Answer from the drawing. Dimensions are ordinates in mm from the lowest x, y and z of the part. Coordinates: 2 decimals unless noted, no trailing zeros. Write each loop counter-clockwise with the first axis right and the second up, starting at its lowest first coordinate (ties: lowest second). Pieces come first, ordered by that corner, then holes. Notation, with made-up numbers: (-37, 5.25) -> (-17, 5.25) arc R12 ccw to (-17, 9.25) -> close; hole circle Ø9 at (52, -19). An arc over 180 degrees is marked (long way). One line per item, written item: value. Start each with the question number.
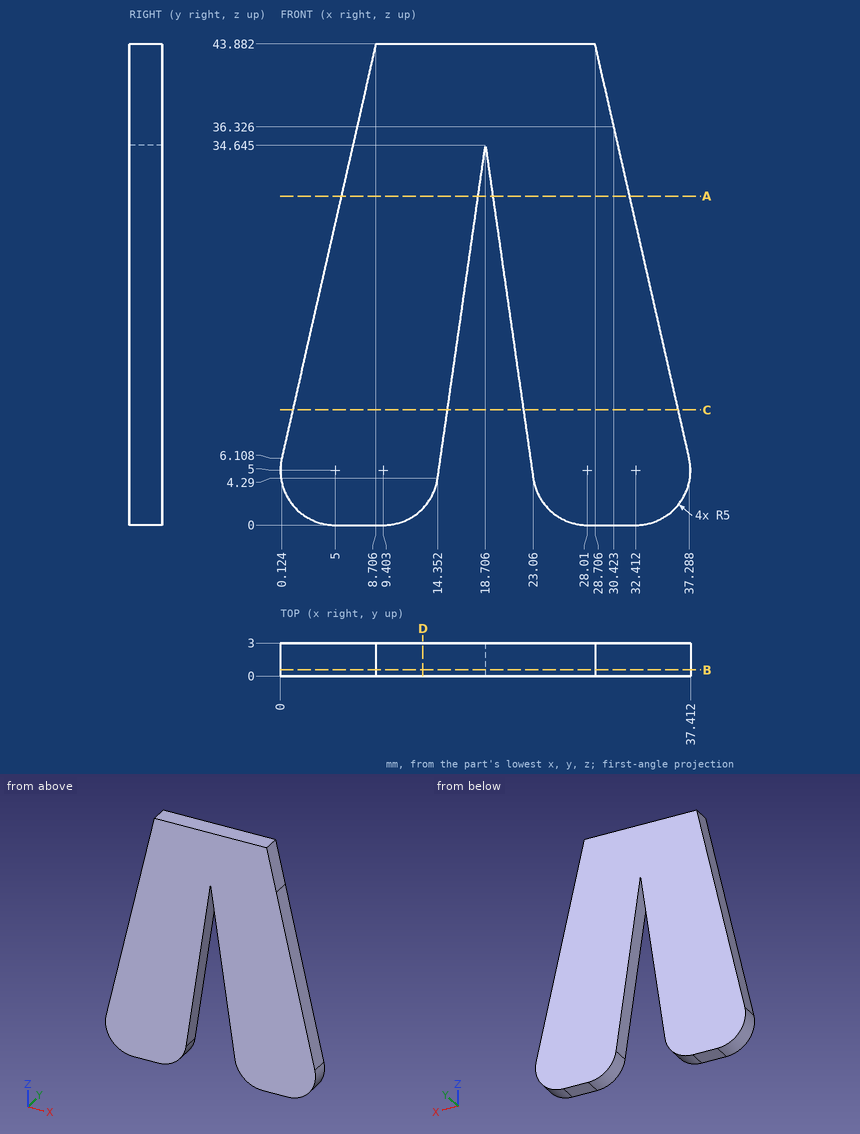
1. Find the intervals of material crossed by probe 1 along X at (y, z) = (1.8, 27); probe 2 along X at (y, z) = (0.9, 14.5) (1 decimal); probe 3 along Z at (x, y) = (23.5, 1.5) (1 decimal), in increasing order. Write a range as from..to.
2. Given pin 1 (1 mm diameter, centred on x = 29, y = 2.5, fed in from +Z), flat-ended and moving along its own axis, determine where the tip first touches the part or whether it passes through.
3. A cutting plane is placed at D-D on x = 13. Give the vertices of the cut face in (y, z).
4. A cutting plane is placed at C-C on z = 10.5. Give the vertices of the cut face in (x, y).
5. A cutting plane is placed at A-A on z = 30. Give the vertices of the cut face in (x, y).
6. A cutting plane is placed at B-B on y = 0.55. Give the vertices of the cut face in (x, z) (1 decimal).
Derived:
1. probe 1: x = 4.87..17.61, 19.8..32.54
1. probe 2: x = 2..15.8, 21.6..35.4
1. probe 3: z = 2.8..43.9
2. pin 1: stops at z = 43.88
3. outline: (0, 1.53) -> (3, 1.53) -> (3, 43.88) -> (0, 43.88) -> close
4. outline: (1.12, 0) -> (15.24, 0) -> (15.24, 3) -> (1.12, 3) -> close; (22.17, 0) -> (36.29, 0) -> (36.29, 3) -> (22.17, 3) -> close
5. outline: (5.55, 0) -> (18.04, 0) -> (18.04, 3) -> (5.55, 3) -> close; (19.37, 0) -> (31.86, 0) -> (31.86, 3) -> (19.37, 3) -> close
6. outline: (0.1, 6.1) arc R5 ccw to (5, 0) -> (9.4, 0) arc R5 ccw to (14.4, 4.3) -> (18.7, 34.6) -> (23.1, 4.3) arc R5 ccw to (28, 0) -> (32.4, 0) arc R5 ccw to (37.3, 6.1) -> (28.7, 43.9) -> (8.7, 43.9) -> close
